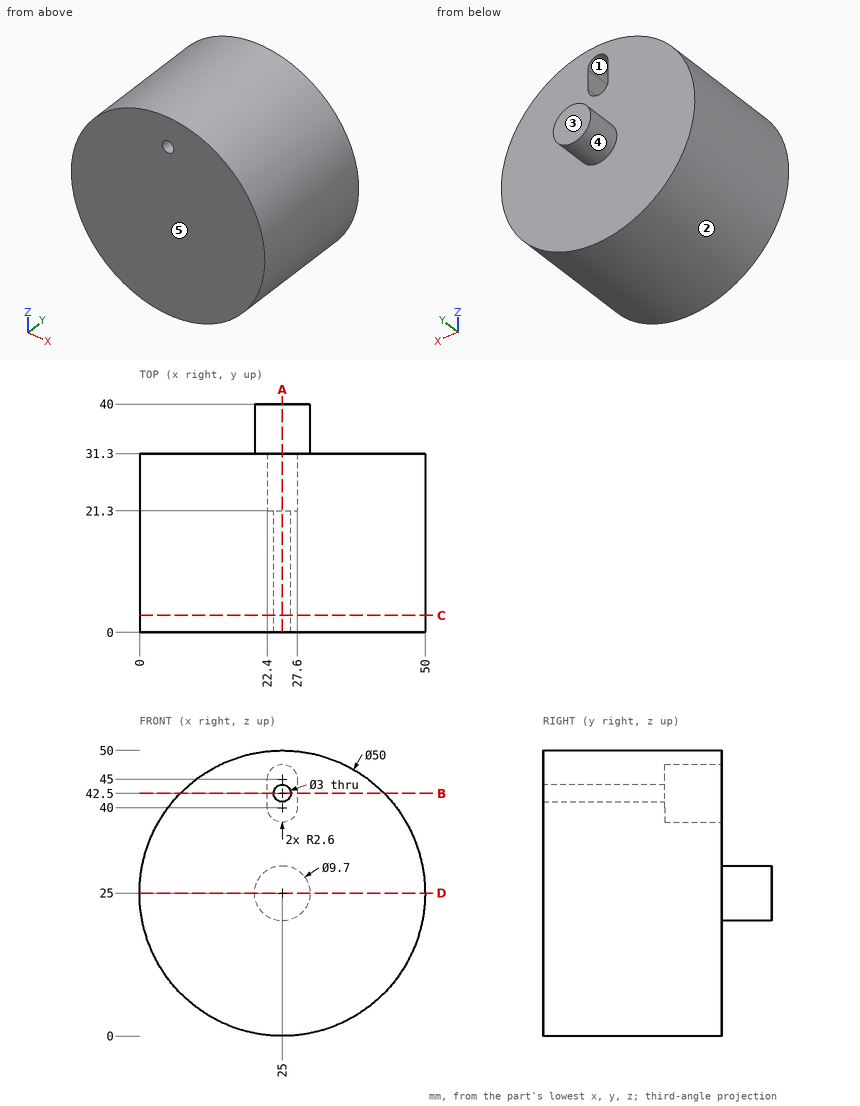
Geometry: see drawing. Coordinates: mm, zero at the bounding-box minimum. A direction names the side the tool comes from. Give positions to 0.01 mm unless a question says otherwise; leave off trailing zeros. Loops run counter-clockwise (first coordinate to the right, second up) from the corner with the lowest first, then second, coordinate; pieces in that order, holes last. Notation, with made-up numbers: (43, -38) - (89, -38) arc R16 ccw to (89, -17) - close; hole circle Ø11 at (76, -19.75). An arc over 180 degrees is marked (long way). One line per question, with ' | ' between items. Start each with the question number.
(1) Section query A-A on x = 25. Return loops of the section in (y, z).
(2) Section query B-B on z = 42.5. Return loops of the section in (x, y).
(3) Pull-direction query (Z, two-part tool) for the marked faces 1, 2 and 3; classes: released by +Z, released by -Z, zero draft, split by the parting line, or undercut.
(4) Contact query for flat-ended pins moving along their axis: pin 1 (4 mm diameter, centred on y = 26, z = 42, fed in from -X); pin 2 (12 mm diameter, centred on x = 33.5, y = 32, fed in from -Z); pin 3 (5 mm diameter, centred on x = 25, z = 42.5, fed in from +Y). Output: stop coordinate, or through.
(5) Section query D-D on z = 25. Return loops of the section in (x, y), then the cut area to 3 significant figures.
(6) Section query C-C on y = 3. Return loops of the section in (x, z).
(7) Ray query, line 1 (Y direction, x = 5, z = 21.5); line 2 (X direction, y = 19, z = 41.5); line 3 (Y direction, x = 26.5, z = 42). Return the intervals inside material, ascending. Write a range as from..to.
(8) Reachability of the marked faces 4 and 5 from +Z, -Z, +X, -X, +Y, -Y: full face, straight path, thin tool, end or side. Return the list, or none.
The answers:
1) outline: (0, 0) - (31.3, 0) - (31.3, 20.15) - (40, 20.15) - (40, 29.85) - (31.3, 29.85) - (31.3, 37.4) - (21.3, 37.4) - (21.3, 41) - (0, 41) - close; (0, 44) - (21.3, 44) - (21.3, 47.6) - (31.3, 47.6) - (31.3, 50) - (0, 50) - close
2) outline: (7.15, 0) - (23.5, 0) - (23.5, 21.3) - (22.4, 21.3) - (22.4, 31.3) - (7.15, 31.3) - close; (26.5, 0) - (42.85, 0) - (42.85, 31.3) - (27.6, 31.3) - (27.6, 21.3) - (26.5, 21.3) - close
3) face 1: undercut | face 2: split by the parting line | face 3: zero draft
4) pin 1: x = 5 | pin 2: z = 0.13 | pin 3: y = 21.3
5) outline: (0, 0) - (50, 0) - (50, 31.3) - (29.85, 31.3) - (29.85, 40) - (20.15, 40) - (20.15, 31.3) - (0, 31.3) - close | area: 1,650 mm2
6) outline: circle Ø50 at (25, 25); hole circle Ø3 at (25, 42.5)
7) line 1: 0..31.3 | line 2: 6.22..23.88, 26.12..43.78 | line 3: 0..21.3
8) face 4: +Y | face 5: +Z, -Z, +X, -X, -Y
